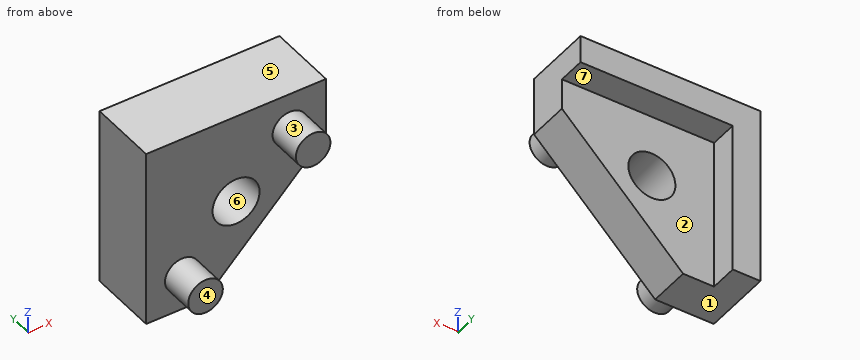
```python
from build123d import *

# Parameters (mm, degrees)
BOSS_EXTRUDE2_DEPTH = 3
SKETCH4_R           = 1.25
BOSS_EXTRUDE3_DEPTH = 2.5
BOSS_EXTRUDE4_DEPTH = 2
CUT_EXTRUDE1_REACH  = 17.835
SKETCH6_R           = 1.7


with BuildPart() as part:
    # Sketch3 → Boss-Extrude2 (new body)
    with BuildSketch(Plane(origin=(0, 0, 0), x_dir=(1, 0, 0), z_dir=(0, 1, 0))):
        Polygon((-2.5, 10.5), (-2.5, -2.5), (10.5, -2.5), (10.5, 1.742640687), (1.742640687, 10.5), align=None)
    extrude(amount=-BOSS_EXTRUDE2_DEPTH)

    # Sketch4 → Boss-Extrude3 (add)
    with BuildSketch(Plane.XZ.offset(3)):
        with Locations(Location((7.889087297, -0.110912703, 0), (0, 0, 90))):
            Circle(SKETCH4_R)
        with Locations(Location((0.110912703, -7.889087297, 0), (0, 0, 90))):
            Circle(SKETCH4_R)
    extrude(amount=BOSS_EXTRUDE3_DEPTH)

    # Sketch5 → Boss-Extrude4 (add)
    with BuildSketch(Plane(origin=(0, 0, 0), x_dir=(1, 0, 0), z_dir=(0, 1, 0))):
        Polygon((-2.5, 10.5), (-2.5, -2.5), (10.5, -2.5), (10.5, -0.5), (-0.5, -0.5), (-0.5, 10.5), align=None)
    extrude(amount=BOSS_EXTRUDE4_DEPTH)

    # Sketch6 → Cut-Extrude1 (cut, up to next)
    with BuildSketch(Plane(origin=(0, 0, 0), x_dir=(1, 0, 0), z_dir=(0, 1, 0)), mode=Mode.PRIVATE) as cut_extrude1_sk1:
        with Locations(Location((4, 4, 0), (0, 0, 270))):
            Circle(SKETCH6_R)
    cut_extrude1_tool1 = extrude(cut_extrude1_sk1.sketch, amount=-CUT_EXTRUDE1_REACH, mode=Mode.PRIVATE) & part.part
    add(cut_extrude1_tool1.solids().sort_by_distance((4, 0, -4))[0], mode=Mode.SUBTRACT)


solid = part.part
```
Model file for the job. Use its own axes, mm. Face numbers are marked on the shaded views. A direction names the side the tool comes from. Round coordinates to 2 decimals unless told otherwise and drop trailing zeros. Write each loop counter-clockwise with the first axis right and the second up, starting at its lowest first coordinate (ties: lowest second). Pieces come first, ordered by that corner, then holes. Notation, with made-up numbers: (41, 88.25) - (60, 88.25) arc R11 ccw to (60, 106.25) - close; hole circle Ø1 at (-31, 5). An arc over 180 degrees is marked (long way). Use CSV: the item, a comma, the result in double quotes. Start each with the question number.
Item 1: Drill centre lines: L1, parallel to Y at x = 2.75, z = -1.75; L2, parallel to X at y = -1.35, z = -4; L3, parallel to Y at x = 0.5, z = -8.25. Where is each one in solid material? Low to high. Write a range as [from, to].
Item 2: Tool access for the marked faces 1, 2 and 3: list every direction of +Z, -Z, +X, -X, +Y, -Y with a clear straight run to the whole face (end or side of a thin tool).
Item 3: Band-saw the part on B-B (z = -4). Write the cut outline in (x, y).
Item 4: Two-plate mould, pull along Z, no slides. Class the marked faces 4, 5, 6 and 7: released by +Z, released by -Z, zero draft, split by the parting line, or undercut.
Item 5: Band-saw the part on D-D (x = 7.5). Write the cut outline in (y, z), and give its area (3 significant figures).
Item 6: Band-saw the part on A-A (x = 5). Write the cut outline in (y, z).
Item 7: Pin check, flat tips, straight feed: P1, Ø1, axis at x = 3.5, y = 1, coming from the -Z side; P2, Ø6.5, axis at x = 1.5, z = -3, coming from the -Y side; P3, Ø3, axis at x = 4, z = -4, coming from the +Y side; P4, Ø0.6, axis at y = 1, z = -5.5, coming from the +X side. Stop position of each tip, or through.
Item 8: Band-saw the part on C-C (y = 0.25). Write the cut outline in (x, z), and give its area (3 significant figures).
Checked values:
1,L1,"y = [-3, 0]"
1,L2,"x = [-2.5, 2.3], [5.7, 8.24]"
1,L3,"y = [-5.5, 0]"
2,face 1,"-Z, +X, -X, +Y, -Y"
2,face 2,"-Z, +X, +Y"
2,face 3,"-Y"
3,outline,"(-2.5, -3) - (2.3, -3) - (2.3, 0) - (-0.5, 0) - (-0.5, 2) - (-2.5, 2) - close; (5.7, -3) - (8.24, -3) - (8.24, 0) - (5.7, 0) - close"
4,face 4,"zero draft"
4,face 5,"released by +Z"
4,face 6,"undercut"
4,face 7,"released by -Z"
5,outline,"(-5.5, -1.3) - (-3, -1.3) - (-3, -4.74) - (0, -4.74) - (0, 0.5) - (2, 0.5) - (2, 2.5) - (-3, 2.5) - (-3, 1.08) - (-5.5, 1.08) - close"
5,area,"31.7 mm²"
6,outline,"(-3, -7.24) - (0, -7.24) - (0, -5.37) - (-3, -5.37) - close; (-3, -2.63) - (0, -2.63) - (0, 0.5) - (2, 0.5) - (2, 2.5) - (-3, 2.5) - close"
7,P1,"stops at z = 0.5"
7,P2,"stops at y = -3"
7,P3,"passes through"
7,P4,"stops at x = -0.5"
8,outline,"(-2.5, -10.5) - (-0.5, -10.5) - (-0.5, 0.5) - (10.5, 0.5) - (10.5, 2.5) - (-2.5, 2.5) - close"
8,area,"48.0 mm²"
